CAD build for the part. Positions are in the model's coordinates, mm. A direction names the side the tool comes from. Round coordinates to 2 decimals unless told otherwise and drop trailing zeros. Write each loop counter-clockwise with the first axis right and the second up, starting at its lowest first coordinate (ties: lowest second). Pieces come first, ordered by that corner, then holes. Notation, with made-up numbers: (22.25, -33.5) -> (40.25, -33.5) arc R8 ccw to (40.25, -26.5) -> close; hole circle Ø8 at (-3.5, 19.5). An arc over 180 degrees is marked (long way). Answer in a Markdown table with one row per item. Add a question column.
```python
from build123d import *

# Parameters (mm, degrees)
SKETCH1_W           = 90
SKETCH1_H           = 80
SKETCH1_W_2         = 35
SKETCH1_H_2         = 60
BOSS_EXTRUDE1_DEPTH = 60
SKETCH2_W           = 46
SKETCH2_H           = 68
CUT_EXTRUDE1_DEPTH  = 58
SKETCH3_W           = 15
SKETCH3_H           = 50
CUT_EXTRUDE2_DEPTH  = 2
SKETCH4_W           = 20
SKETCH4_H           = 20
CUT_EXTRUDE3_DEPTH  = 10
SKETCH5_W           = 55
SKETCH5_H           = 60
CUT_EXTRUDE4_DEPTH  = 10


with BuildPart() as part:
    # Sketch1 → Boss-Extrude1 (new body)
    with BuildSketch(Plane(origin=(0, 0, 0), x_dir=(1, 0, 0), z_dir=(0, 1, 0))):
        with Locations((-5.196940727, -10.728489484)):
            Rectangle(SKETCH1_W, SKETCH1_H)
        with Locations((17.303059273, -10.728489484)):
            Rectangle(SKETCH1_W_2, SKETCH1_H_2, mode=Mode.SUBTRACT)
    extrude(amount=BOSS_EXTRUDE1_DEPTH)

    # Sketch2 → Cut-Extrude1 (cut)
    with BuildSketch(Plane(origin=(0, 60, 0), x_dir=(1, 0, 0), z_dir=(0, 1, 0))):
        with Locations((-25.196940727, -6.728489484)):
            Rectangle(SKETCH2_W, SKETCH2_H)
    extrude(amount=-CUT_EXTRUDE1_DEPTH, mode=Mode.SUBTRACT)

    # Sketch3 → Cut-Extrude2 (cut)
    with BuildSketch(Plane.ZY.offset(2.196940727)):
        with Locations((25.228489484, 35)):
            Rectangle(SKETCH3_W, SKETCH3_H)
    extrude(amount=-CUT_EXTRUDE2_DEPTH, mode=Mode.SUBTRACT)

    # Sketch4 → Cut-Extrude3 (cut)
    with BuildSketch(Plane(origin=(0, 0, -29.271510516), x_dir=(-1, 0, 0), z_dir=(0, 0, -1))):
        with Locations((-24.803059273, 50)):
            Rectangle(SKETCH4_W, SKETCH4_H)
    extrude(amount=-CUT_EXTRUDE3_DEPTH, mode=Mode.SUBTRACT)

    # Sketch5 → Cut-Extrude4 (cut)
    with BuildSketch(Plane(origin=(39.803059273, 0, 0), x_dir=(0, 0, -1), z_dir=(1, 0, 0))):
        with Locations((-10.728489484, 30)):
            Rectangle(SKETCH5_W, SKETCH5_H)
    extrude(amount=-CUT_EXTRUDE4_DEPTH, mode=Mode.SUBTRACT)

    # Sketch14 → CSK for M3 Flat Head Machine Screw1 (revolve, cut)
    with BuildSketch(Plane(origin=(-5.196940727, 30, -29.271510516), x_dir=(0, 1, 0), z_dir=(1, 0, 0))):
        Polygon((0, 0), (0, 3.081549114), (1.8, 2), (1.8, 1.35), (3.15, 0), align=None)
    revolve(axis=Axis((-5.196940727, 30, -35.621510516), (0, 0, 1)), mode=Mode.SUBTRACT)


solid = part.part
```
Item 1: Two-plate mould, pull along X, no slides. Class faces 1 (the flat face through (-6, 23, -29.272)), 2 (the flat face through (-50.197, 30, 11)), 3 (the flat face through (25, 40, -24)), 4 (the flat face through (39.803, 30, 45)): +X half, -X half, draft (parallel to the pull), parting line (faces both ways), or undercut.
Item 2: Tool access for faces 5 (the flat face through (-26, 2, 6)), 6 (the flat face through (14.803, 50, -24)), 7 (the flat face through (37, 30, -16.772)): list every direction of +Z, -Z, +X, -X, +Y, -Y with a clear straight run to the whole face (end or side of a thin tool).
Item 3: Saw through at B-B on y = 5.5. Give the cut face in (x, z), then the cut area to 3 significant figures.
Item 4: Saw through at C-C on z = 12.5. Give the cut face in (x, y).
Item 5: Saw through at D-D on y = 17.5. Give the cut face in (x, z), then the cut area to 3 significant figures.
Item 6: Drill centre lines: probe 1 along X at (y, z) = (49, -18); probe 2 along Z at (x, y) = (-31, 57); probe 3 along Z at (x, y) = (-0.5, 54). Where is each one in solid material? Low to high.
Item 7: Saw through at A-A on y = 55. Give the cut face in (x, z), then the cut area to 3 significant figures.
Item 8: Pin check, flat tips, straight feed: pin 1 (1.5 mm diameter, centred on y = 18.5, z = 1, fed in from +X); pin 2 (3 mm diameter, centred on x = -7, z = 22.5, fed in from +Y); pin 3 (1 mm diameter, centred on y = 33.5, z = 26.5, fed in from +X). Stop position of each tip, or through.
Recorded:
| question | item | result |
|---|---|---|
| 1 | face 1 | draft |
| 1 | face 2 | -X half |
| 1 | face 3 | undercut |
| 1 | face 4 | +X half |
| 2 | face 5 | +Y |
| 2 | face 6 | -Z, +Y |
| 2 | face 7 | +X, +Y, -Y |
| 3 | outline | (-50.2, -29.27) -> (39.8, -29.27) -> (39.8, -16.77) -> (34.8, -16.77) -> (34.8, -19.27) -> (-0.2, -19.27) -> (-0.2, 40.73) -> (34.8, 40.73) -> (34.8, 38.23) -> (39.8, 38.23) -> (39.8, 50.73) -> (-50.2, 50.73) -> close; hole (-48.2, -27.27) -> (-2.2, -27.27) -> (-2.2, 40.73) -> (-48.2, 40.73) -> close |
| 3 | area | 1,700 mm2 |
| 4 | outline | (-50.2, 0) -> (-0.2, 0) -> (-0.2, 60) -> (-2.2, 60) -> (-2.2, 2) -> (-48.2, 2) -> (-48.2, 60) -> (-50.2, 60) -> close |
| 5 | outline | (-50.2, -29.27) -> (39.8, -29.27) -> (39.8, -16.77) -> (34.8, -16.77) -> (34.8, -19.27) -> (-0.2, -19.27) -> (-0.2, 17.73) -> (-2.2, 17.73) -> (-2.2, -27.27) -> (-48.2, -27.27) -> (-48.2, 40.73) -> (-2.2, 40.73) -> (-2.2, 32.73) -> (-0.2, 32.73) -> (-0.2, 40.73) -> (34.8, 40.73) -> (34.8, 38.23) -> (39.8, 38.23) -> (39.8, 50.73) -> (-50.2, 50.73) -> close |
| 5 | area | 1,670 mm2 |
| 6 | probe 1 | -50.2 to -48.2, -2.2 to -0.2, 34.8 to 39.8 |
| 6 | probe 2 | -29.27 to -27.27, 40.73 to 50.73 |
| 6 | probe 3 | -29.27 to 17.73, 32.73 to 50.73 |
| 7 | outline | (-50.2, -29.27) -> (14.8, -29.27) -> (14.8, -19.27) -> (-0.2, -19.27) -> (-0.2, 17.73) -> (-2.2, 17.73) -> (-2.2, -27.27) -> (-48.2, -27.27) -> (-48.2, 40.73) -> (-2.2, 40.73) -> (-2.2, 32.73) -> (-0.2, 32.73) -> (-0.2, 40.73) -> (34.8, 40.73) -> (34.8, 38.23) -> (39.8, 38.23) -> (39.8, 50.73) -> (-50.2, 50.73) -> close; (34.8, -29.27) -> (39.8, -29.27) -> (39.8, -16.77) -> (34.8, -16.77) -> close |
| 7 | area | 1,470 mm2 |
| 8 | pin 1 | x = -0.2 |
| 8 | pin 2 | y = 2 |
| 8 | pin 3 | x = -48.2 |
